Build history of the part. All positions in model axes, mm. Face numbers are marked on the shaded views. A direction names the side the tool comes from. Give positions to 0.01 mm unless a question says otherwise; leave off trailing zeros. Order: outer loops, then holes, each group sorted by start corner. A loop starts at its lowest first (then second) coordinate and runs counter-clockwise, first axis right, second up. Notation, with made-up numbers: (49.5, 33.5) - (77.5, 33.5) arc R14 ccw to (77.5, 46.5) - close; hole circle Ø5 at (76, 10.5). An arc over 180 degrees is marked (long way). Write each question's results on one line, items separated by ' | '. Start each with the question number.
1) Cut at B-B on y = -23.6. List the corners of the cut face in (x, z), plus the area to 3 significant figures.
2) Cut at A-A on x = -48. List the corners of the cut face in (y, z).
3) Two-plate mould, pull along Y, no slides. Class the marked faces 1 and 2: +Y half, -Y half, draft (parallel to the pull), parting line (faces both ways), or undercut.
4) Cut at C-C on y = -18.6. List the corners of the cut face in (x, z), plus the area to 3 significant figures.
5) Drill centre lines: line 1 along X through (y, z) = (-25.5, 0.75); line 2 along Y through (x, z) = (-89.9, 1.1); line 3 along Y through (x, z) = (-38.5, 1.65). Where is each one in solid material? Low to high. Write a range as from..to.
6) Cut at D-D on x = 0. List the corners of the cut face in (y, z), plus the area to 3 significant figures.
7) Drop flat-ended pins along their axis: pin 1 Ø1 at (x, z) = (2.5, 1.5) entering from -Y; pin 2 Ø0.6 at (y, z) = (-19.5, 1) entering from +X; pin 3 Ø11.5 at (x, y) = (-43.5, -28.5) entering from +Z. Give the stop position or say it passes through.
8) Tool access for the marked faces 3 and 4: list every direction of +Z, -Z, +X, -X, +Y, -Y with a clear straight run to the whole face (end or side of a thin tool).
from build123d import *

# Parameters (mm, degrees)
SKETCH_R        = 1.7
PAD_DEPTH       = 3
SKETCH001_W     = 105.5
SKETCH001_H     = 23
POCKET_DEPTH    = 1
SKETCH002_R     = 1.2
SKETCH002_W     = 54
SKETCH002_H     = 13.5
SKETCH002_W_2   = 19
SKETCH002_H_2   = 13.4
POCKET001_DEPTH = 5
FILLET_R        = 5
FILLET001_R     = 5
FILLET002_R     = 5
FILLET003_R     = 5
SKETCH003_W     = 14
SKETCH003_H     = 8
POCKET002_DEPTH = 5
SKETCH004_R     = 11
PAD001_DEPTH    = 3
SKETCH005_R     = 10.1
POCKET003_DEPTH = 5.1


with BuildPart() as part:
    # Sketch → Pad (new body)
    with BuildSketch(Plane.XY):
        Polygon((-12.902803, 11.999952), (12.501955, 11.999952), (12.475984, 5), (22.475984, 5), (22.475984, -5), (12.5, -5), (12.5, -12), (12.5, -37), (-97.5, -37), (-97.5, 11.999952), align=None)
        with Locations((17.475984, 0)):
            Circle(SKETCH_R, mode=Mode.SUBTRACT)
        with Locations((-92.5, 0)):
            Circle(SKETCH_R, mode=Mode.SUBTRACT)
        with Locations((-25, 0)):
            Circle(SKETCH_R, mode=Mode.SUBTRACT)
    extrude(amount=PAD_DEPTH)

    # Sketch001 (on Face15 of Pad) → Pocket (cut)
    with BuildSketch(Plane.XY.offset(3)):
        with Locations((-42.25, -24)):
            Rectangle(SKETCH001_W, SKETCH001_H)
    extrude(amount=-POCKET_DEPTH, mode=Mode.SUBTRACT)

    # Sketch002 (on Face20 of Pocket) → Pocket001 (cut)
    with BuildSketch(Plane.XY.offset(2)):
        with Locations((-89.9, -18.6)):
            Circle(SKETCH002_R)
        with Locations((-89.9, -30.6)):
            Circle(SKETCH002_R)
        with Locations((-24.8, -18.6)):
            Circle(SKETCH002_R)
        with Locations((5.4, -23.6)):
            Circle(SKETCH002_R)
        with Locations((-58.2, -21.55)):
            Rectangle(SKETCH002_W, SKETCH002_H)
        with Locations((-8, -20.8)):
            Rectangle(SKETCH002_W_2, SKETCH002_H_2)
    extrude(amount=-POCKET001_DEPTH, mode=Mode.SUBTRACT)

    # Fillet
    fillet_edges = [part.edges().sort_by_distance(p)[0] for p in [
        (10.5, -35.5, 2.5),
    ]]
    fillet(fillet_edges, radius=FILLET_R)

    # Fillet001
    fillet001_edges = [part.edges().sort_by_distance(p)[0] for p in [
        (-95, -35.5, 2.5),
    ]]
    fillet(fillet001_edges, radius=FILLET001_R)

    # Fillet002
    fillet002_edges = [part.edges().sort_by_distance(p)[0] for p in [
        (-97.5, -37, 1.5),
    ]]
    fillet(fillet002_edges, radius=FILLET002_R)

    # Fillet003
    fillet003_edges = [part.edges().sort_by_distance(p)[0] for p in [
        (12.5, -37, 1.5),
    ]]
    fillet(fillet003_edges, radius=FILLET003_R)

    # Sketch003 (on Face1 of Fillet003) → Pocket002 (cut)
    with BuildSketch(Plane.XY.offset(3)):
        with Locations((-0.6, -33)):
            Rectangle(SKETCH003_W, SKETCH003_H)
    extrude(amount=-POCKET002_DEPTH, mode=Mode.SUBTRACT)

    # Sketch004 (on Face26 of Pocket002) → Pad001 (join)
    with BuildSketch(Plane(origin=(0, 0, 0), x_dir=(1, 0, 0), z_dir=(0, 0, -1))):
        Circle(SKETCH004_R)
    extrude(amount=PAD001_DEPTH)

    # Sketch005 (on Face1 of Pad001) → Pocket003 (cut)
    with BuildSketch(Plane.XY.offset(3)):
        Circle(SKETCH005_R)
    extrude(amount=-POCKET003_DEPTH, mode=Mode.SUBTRACT)


solid = part.part
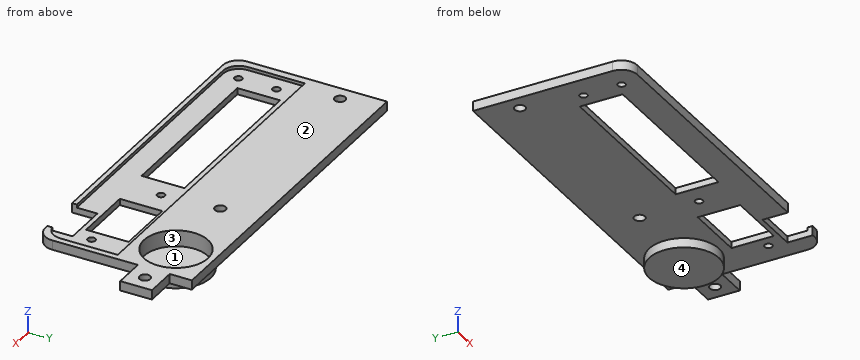
Results:
1) outline: (-97.5, 0) - (-85.2, 0) - (-85.2, 2) - (-95, 2) - (-95, 3) - (-97.5, 3) - close; (-31.2, 0) - (-17.5, 0) - (-17.5, 2) - (-31.2, 2) - close; (1.5, 0) - (4.2, 0) - (4.2, 2) - (1.5, 2) - close; (6.6, 0) - (12.5, 0) - (12.5, 3) - (10.5, 3) - (10.5, 2) - (6.6, 2) - close | area: 73.7 mm^2
2) outline: (-37, 0) - (-28.3, 0) - (-28.3, 2) - (-35.5, 2) - (-35.5, 3) - (-37, 3) - close; (-14.8, 0) - (12, 0) - (12, 3) - (-12.5, 3) - (-12.5, 2) - (-14.8, 2) - close
3) face 1: undercut | face 2: draft
4) outline: (-97.5, 0) - (-91.1, 0) - (-91.1, 2) - (-95, 2) - (-95, 3) - (-97.5, 3) - close; (-88.7, 0) - (-85.2, 0) - (-85.2, 2) - (-88.7, 2) - close; (-31.2, 0) - (-26, 0) - (-26, 2) - (-31.2, 2) - close; (-23.6, 0) - (-17.5, 0) - (-17.5, 2) - (-23.6, 2) - close; (1.5, 0) - (12.5, 0) - (12.5, 3) - (10.5, 3) - (10.5, 2) - (1.5, 2) - close | area: 68.9 mm^2
5) line 1: -97.5..-85.2, -31.2..-17.5, 1.5..12.5 | line 2: -37..-31.8, -29.4..-19.8, -17.4..12 | line 3: -37..-28.3, -14.8..12
6) outline: (-29, 0) - (-27.5, 0) - (-27.5, 2) - (-29, 2) - close; (-14.1, 0) - (-11, 0) - (-11, -3) - (11, -3) - (11, 0) - (12, 0) - (12, 3) - (10.1, 3) - (10.1, -2.1) - (-10.1, -2.1) - (-10.1, 3) - (-12.5, 3) - (-12.5, 2) - (-14.1, 2) - close | area: 42.7 mm^2
7) pin 1: y = -29 | pin 2: x = 12.5 | pin 3: z = 2
8) face 3: +Z | face 4: -Z, +X, -X, +Y, -Y
